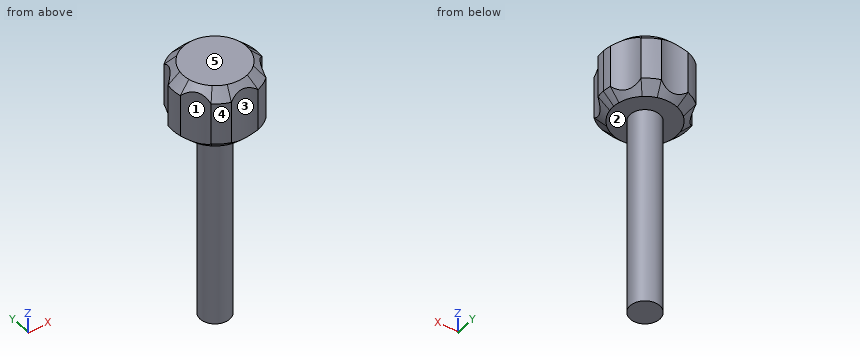
from build123d import *

# Parameters (mm, degrees)
F0_R     = 1.4
F1_DEPTH = 6
F2_SIZE  = 1
F3_DEPTH = 6.001
F4_DEPTH = 19


with BuildPart() as f1:
    # F0 (on Top) → F1 (new body)
    with BuildSketch(Plane.XY):
        with BuildLine():
            ThreePointArc((3.9226903411, -0.7826241038), (3.9806256647, -0.3932166296), (4, 0))
            ThreePointArc((4, 0), (3.9806256647, 0.3932166296), (3.9226903411, 0.7826241038))
            ThreePointArc((3.9226903411, 0.7826241038), (3.0310889132, 1.75), (2.639117526, 3.0058374347))
            ThreePointArc((2.639117526, 3.0058374347), (2, 3.4641016151), (1.2835728151, 3.7884615385))
            ThreePointArc((1.2835728151, 3.7884615385), (0, 3.5), (-1.2835728151, 3.7884615385))
            ThreePointArc((-1.2835728151, 3.7884615385), (-2, 3.4641016151), (-2.639117526, 3.0058374347))
            ThreePointArc((-2.639117526, 3.0058374347), (-3.0310889132, 1.75), (-3.9226903411, 0.7826241038))
            ThreePointArc((-3.9226903411, 0.7826241038), (-4, 0), (-3.9226903411, -0.7826241038))
            ThreePointArc((-3.9226903411, -0.7826241038), (-3.0310889132, -1.75), (-2.639117526, -3.0058374347))
            ThreePointArc((-2.639117526, -3.0058374347), (-2, -3.4641016151), (-1.2835728151, -3.7884615385))
            ThreePointArc((-1.2835728151, -3.7884615385), (0, -3.5), (1.2835728151, -3.7884615385))
            ThreePointArc((1.2835728151, -3.7884615385), (2, -3.4641016151), (2.639117526, -3.0058374347))
            ThreePointArc((2.639117526, -3.0058374347), (3.0310889132, -1.75), (3.9226903411, -0.7826241038))
        make_face()
        Circle(F0_R, mode=Mode.SUBTRACT)
        Circle(F0_R)
        with BuildLine():
            ThreePointArc((-1.2835728151, 3.7884615385), (0, 3.5), (1.2835728151, 3.7884615385))
            ThreePointArc((1.2835728151, 3.7884615385), (0, 4), (-1.2835728151, 3.7884615385))
        make_face()
        with BuildLine():
            ThreePointArc((2.639117526, 3.0058374347), (3.0310889132, 1.75), (3.9226903411, 0.7826241038))
            ThreePointArc((3.9226903411, 0.7826241038), (3.4641016151, 2), (2.639117526, 3.0058374347))
        make_face()
        with BuildLine():
            ThreePointArc((2.639117526, -3.0058374347), (3.4641016151, -2), (3.9226903411, -0.7826241038))
            ThreePointArc((3.9226903411, -0.7826241038), (3.0310889132, -1.75), (2.639117526, -3.0058374347))
        make_face()
        with BuildLine():
            ThreePointArc((-1.2835728151, -3.7884615385), (0, -4), (1.2835728151, -3.7884615385))
            ThreePointArc((1.2835728151, -3.7884615385), (0, -3.5), (-1.2835728151, -3.7884615385))
        make_face()
        with BuildLine():
            ThreePointArc((-3.9226903411, -0.7826241038), (-3.4641016151, -2), (-2.639117526, -3.0058374347))
            ThreePointArc((-2.639117526, -3.0058374347), (-3.0310889132, -1.75), (-3.9226903411, -0.7826241038))
        make_face()
        with BuildLine():
            ThreePointArc((-3.9226903411, 0.7826241038), (-3.0310889132, 1.75), (-2.639117526, 3.0058374347))
            ThreePointArc((-2.639117526, 3.0058374347), (-3.4641016151, 2), (-3.9226903411, 0.7826241038))
        make_face()
    extrude(amount=F1_DEPTH)

    # F2
    f2_edges = [f1.edges().sort_by_distance(p)[0] for p in [
        (2.639118, -3.005837, 6),
        (2.639118, -3.005837, 0),
    ]]
    chamfer(f2_edges, length=F2_SIZE)

    # F0 (on Top) → F3 (cut, through all)
    with BuildSketch(Plane.XY):
        with BuildLine():
            ThreePointArc((-1.2835728151, -3.7884615385), (0, -4), (1.2835728151, -3.7884615385))
            ThreePointArc((1.2835728151, -3.7884615385), (0, -3.5), (-1.2835728151, -3.7884615385))
        make_face()
        with BuildLine():
            ThreePointArc((-3.9226903411, -0.7826241038), (-3.4641016151, -2), (-2.639117526, -3.0058374347))
            ThreePointArc((-2.639117526, -3.0058374347), (-3.0310889132, -1.75), (-3.9226903411, -0.7826241038))
        make_face()
        with BuildLine():
            ThreePointArc((2.639117526, -3.0058374347), (3.4641016151, -2), (3.9226903411, -0.7826241038))
            ThreePointArc((3.9226903411, -0.7826241038), (3.0310889132, -1.75), (2.639117526, -3.0058374347))
        make_face()
        with BuildLine():
            ThreePointArc((2.639117526, 3.0058374347), (3.0310889132, 1.75), (3.9226903411, 0.7826241038))
            ThreePointArc((3.9226903411, 0.7826241038), (3.4641016151, 2), (2.639117526, 3.0058374347))
        make_face()
        with BuildLine():
            ThreePointArc((-1.2835728151, 3.7884615385), (0, 3.5), (1.2835728151, 3.7884615385))
            ThreePointArc((1.2835728151, 3.7884615385), (0, 4), (-1.2835728151, 3.7884615385))
        make_face()
        with BuildLine():
            ThreePointArc((-3.9226903411, 0.7826241038), (-3.0310889132, 1.75), (-2.639117526, 3.0058374347))
            ThreePointArc((-2.639117526, 3.0058374347), (-3.4641016151, 2), (-3.9226903411, 0.7826241038))
        make_face()
    extrude(amount=F3_DEPTH, mode=Mode.SUBTRACT)

    # F0 (on Top) → F4 (join)
    with BuildSketch(Plane.XY):
        Circle(F0_R)
    extrude(amount=-F4_DEPTH)


solid = f1.part
CAD build for the part. Positions are in the model's coordinates, mm. Face numbers are marked on the shaded views. A direction names the side the tool comes from. Give positions to 0.01 mm unless a question says otherwise; leave off trailing zeros. Write each loop counter-clockwise with the first axis right and the second up, starting at its lowest first coordinate (ties: lowest second). Pieces come first, ordered by that corner, then holes. Notation, with made-up numbers: M 24.25,50.5 L 29.25,50.5 A12 ccw 29.25,61.5 Z; hole C 28.25,-29.75 d2. An arc over 180 degrees is marked long. Put each result on its own line as item: value. Start each with the question number.
(1) Probe L1, parallel to Z at x = -0.5, y = 2.75; L2, parallel to Y at x = 0, z = -12.5; L3, parallel to X at y = 0.75, z = 2.25. List the from-to ranges inside material, lowest first.
(2) Mould opens along X. For the marked faces 3, 4 and 5 say: +X half, -X half, draft (parallel to the pull), parting line (faces both ways), or undercut.
(3) Flat gauge pins, fed straight in: pin 1 Ø1 at (y, z) = (-2.5, 0.5) entering from +X; pin 2 Ø3 at (y, z) = (-2, -12.5) entering from -X; pin 3 Ø3 at (y, z) = (-1.5, -15) entering from +X. Where does each tip first touch, or does it go through?
(4) Band-saw the part on B-B, the plane z = -15. Write the cut outline in (x, y), and give its area (3 significant figures).
(5) Band-saw the part on A-A, the plane x = 0. Write the cut outline in (y, z), and give its area (3 significant figures).
(6) Which spindle directions (+Z, -Z, +X, -X, +Y, -Y) get a long thin tool onto all of the face, cutting with end or side? Do the marked faces 1 and 2. Say none if no direction does.
Response values:
1. L1: z = 0 to 6
1. L2: y = -1.4 to 1.4
1. L3: x = -3.93 to 3.93
2. face 3: undercut
2. face 4: -X half
2. face 5: draft
3. pin 1: stops at x = 2.9
3. pin 2: stops at x = -1.31
3. pin 3: stops at x = 1.4
4. outline: C 0,0 d2.8
4. area: 6.16 mm2
5. outline: M -3.5,0.5 L -3,0 L -1.4,0 L -1.4,-19 L 1.4,-19 L 1.4,0 L 3,0 L 3.5,0.5 L 3.5,5.5 L 3,6 L -3,6 L -3.5,5.5 Z
5. area: 94.7 mm2
6. face 1: +Z, -Z, -X, -Y
6. face 2: -Z
